Read the model definition and answer for the solid it produces. Units are mm, in the model's axes. Face numbers are marked on the shaded views. Coordinates: 2 decimals unless noted, no trailing zeros. Loops run counter-clockwise (first coordinate to the right, second up) from the corner with the lowest first, then second, coordinate; pieces in that order, holes last. Notation, with made-up numbers: (59.5, 21.25) -> (92.5, 21.25) arc R18 ccw to (92.5, 34.25) -> close; hole circle Ø3 at (-34, 78). An arc over 180 degrees is marked (long way). Answer as a JSON object with one key per item and string values. Group by question number.
1) Flat-ended cylindrical pins translate along their axes: P1, Ø0.8, axis at x = -249.5, y = 0.5, coming from the -Z side; P2, Ø0.8, axis at y = 1, z = 460.5, coming from the +X side; P3, Ø0.8, axis at x = -249.5, y = 1, coming from the +Z side. Find the tip coordinate at first contact, or state that the pin passes through.
2) Determine the mould class of the marked faces 1, 2 and 3 for opening direction X: released by +X, released by -X, zero draft, split by the parting line, or undercut.
3) Section D-D, the plane z = 469 is taken. Give the vertices of the cut face in (x, y), plus the area to 3 significant figures.
4) Section C-C, the plane x = -274.5 is taken. Give the vertices of the cut face in (y, z).
5) Section B-B, the plane y = 0.6 is taken. Give the vertices of the cut face in (x, z).
6) Consider probe 1 along X at (y, z) = (1.2, 464.75); probe 2 along X at (y, z) = (0.6, 466.25); probe 3 along Z at (x, y) = (-274, 0.3). Determine where each line is inside the solid, lowest interval first. Write a range as [from, to].
7) Section A-A, the plane z = 466.75 is taken. Give the vertices of the cut face in (x, y), plus the area to 3 significant figures.
Autodesk Inventor part; units mm, degrees
ref_plane "YZ Plane" through (0, 0, 0) normal (1, 0, 0) x (0, 1, 0)
ref_plane "XZ Plane" through (0, 0, 0) normal (0, 1, 0) x (-1, 0, 0)
ref_plane "XY Plane" through (0, 0, 0) normal (0, 0, 1) x (1, 0, 0)
sketch "Sketch1" plane through (0, 0, 0) normal (0, 1, 0) x (-1, 0, 0)
  line L0 (270.588, 471.9828) -> (250.588, 471.9828)
  line L1 (250.588, 459.4828) -> (270.588, 459.4828)
  line L2 (276.588, 465.4828) -> (276.588, 465.9828)
  arc A0 (276.588, 465.9828) -> (270.588, 471.9828) centre (270.588, 465.9828) ccw
  arc A1 (270.588, 459.4828) -> (276.588, 465.4828) centre (270.588, 465.4828) ccw
  circle A2 centre (270.588, 465.7328) radius 1.75
  line L3 (250.588, 459.4828) -> (250.588, 461.4828)
  line L4 (250.588, 461.4828) -> (248.588, 461.4828)
  line L5 (248.588, 462.9828) -> (250.588, 462.9828)
  line L6 (250.588, 462.9828) -> (250.588, 464.9828)
  line L7 (250.588, 464.9828) -> (248.588, 464.9828)
  line L8 (248.588, 466.4828) -> (250.588, 466.4828)
  line L9 (250.588, 466.4828) -> (250.588, 468.4828)
  line L10 (250.588, 468.4828) -> (248.588, 468.4828)
  line L11 (248.588, 462.9828) -> (248.588, 461.4828)
  line L12 (248.588, 469.9828) -> (248.588, 468.4828)
  line L13 (248.588, 466.4828) -> (248.588, 464.9828)
  line L14 (248.588, 469.9828) -> (250.588, 469.9828)
  line L15 (250.588, 469.9828) -> (250.588, 471.9828)
  point P0 (0, 0)
  point P1 (276.588, 471.9828)
  point P2 (276.588, 459.4828)
  dimension "d2" = 6
  dimension "d5" = 3.5
  dimension "d15" = 0
  dimension "d26" = 2
  dimension "d27" = 2
  dimension "d28" = 2
  dimension "d29" = 2
  dimension "d30" = 2
  dimension "d31" = 2
  dimension "d32" = 1.5
  dimension "d33" = 1.5
  dimension "d34" = 2
  dimension "d35" = 1.5
  dimension "d36" = 2
  dimension "d39" = 20
extrude "Extrusion7" add sketch "Sketch1" along normal blind 1.524
properties part number "Connection4-3.5"
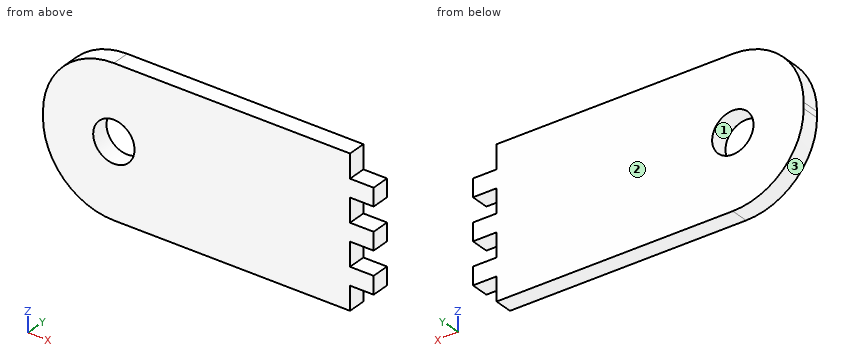
Determined:
{
 "1": {"P1": "z = 461.48", "P2": "x = -250.59", "P3": "z = 469.98"},
 "2": {"face 1": "undercut", "face 2": "zero draft", "face 3": "released by -X"},
 "3": {"outline": "(-275.77, 0) -> (-248.59, 0) -> (-248.59, 1.52) -> (-275.77, 1.52) -> close", "area": "41.4 mm²"},
 "4": {"outline": "(0, 460.93) -> (1.52, 460.93) -> (1.52, 470.53) -> (0, 470.53) -> close"},
 "5": {"outline": "(-276.59, 465.48) arc R6 ccw to (-270.59, 459.48) -> (-250.59, 459.48) -> (-250.59, 461.48) -> (-248.59, 461.48) -> (-248.59, 462.98) -> (-250.59, 462.98) -> (-250.59, 464.98) -> (-248.59, 464.98) -> (-248.59, 466.48) -> (-250.59, 466.48) -> (-250.59, 468.48) -> (-248.59, 468.48) -> (-248.59, 469.98) -> (-250.59, 469.98) -> (-250.59, 471.98) -> (-270.59, 471.98) arc R6 ccw to (-276.59, 465.98) -> close; hole circle Ø3.5 at (-270.59, 465.73)"},
 "6": {"probe 1": "[-276.54, -272.04], [-269.14, -250.59]", "probe 2": "[-276.58, -272.26], [-268.92, -248.59]", "probe 3": "[460.55, 470.92]"},
 "7": {"outline": "(-276.54, 0) -> (-272.01, 0) -> (-272.01, 1.52) -> (-276.54, 1.52) -> close; (-269.16, 0) -> (-250.59, 0) -> (-250.59, 1.52) -> (-269.16, 1.52) -> close", "area": "35.2 mm²"}
}
